Source: three-view drawing plus pictorial views. Frame: mm from the lowest corner of the part. Give positions to 0.01 mm unless a question says otherwise; leave off trailing zeros. Loops run counter-clockwise (first coordinate to the right, second up) from the corner with the lowest first, then second, coordinate; pieces in that order, holes last. Notation, with made-up numbers: (45.25, 87) - (87.25, 87) arc R17 ccw to (87.25, 120) - close; hole circle Ø4 at (54.5, -17.5). An arc over 180 degrees is marked (long way). Answer as a JSON object with one key per item and string values. Group by question number.
(1) Material intervals for L1, parallel to Z at x = 5, y = 2.75; L2, parallel to X at y = 2.1, z = 12, sorted ascending.
(2) Section query C-C (y = 2.8). Return loops of the section in (x, z), plus the area to 3 significant figures.
(3) Section query B-B (x = 5). Return loops of the section in (y, z).
(4) Section query A-A (z = 18). Return loops of the section in (x, y), plus the area to 3 significant figures.
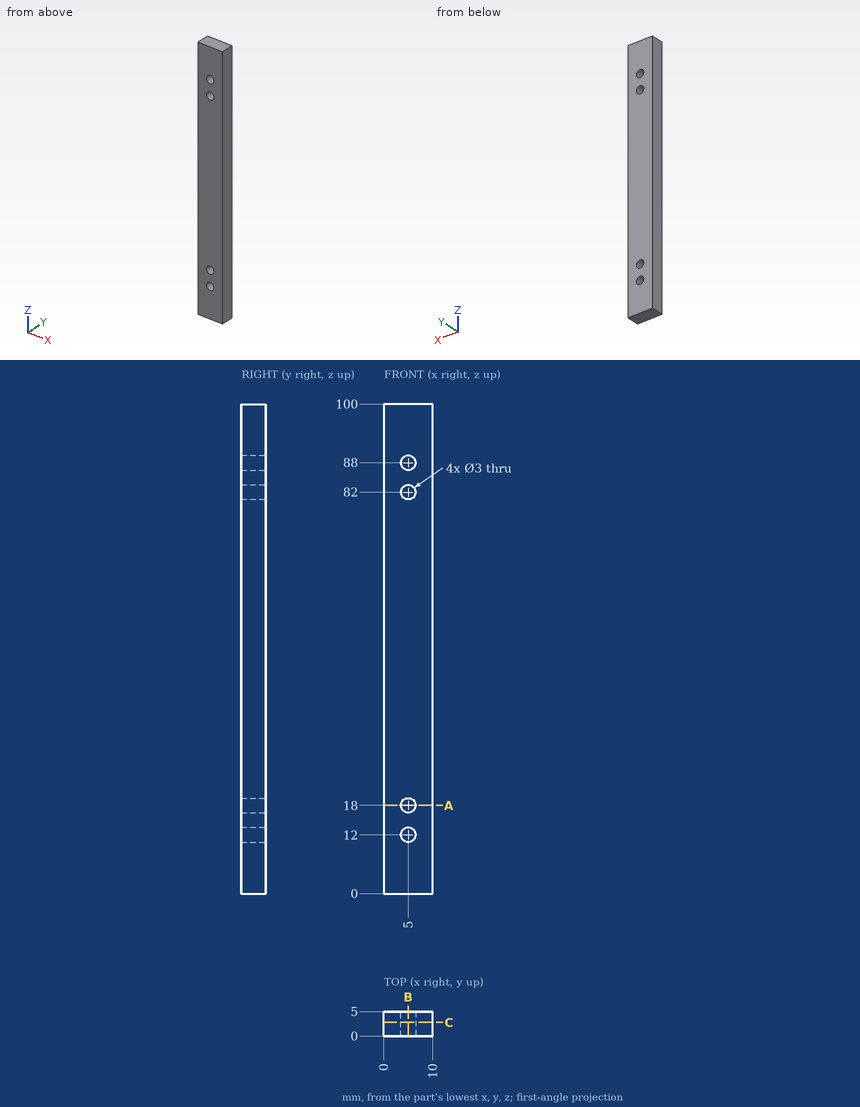
Recorded:
{
 "1": {"L1": "z = 0 to 10.5, 13.5 to 16.5, 19.5 to 80.5, 83.5 to 86.5, 89.5 to 100", "L2": "x = 0 to 3.5, 6.5 to 10"},
 "2": {"outline": "(0, 0) - (10, 0) - (10, 100) - (0, 100) - close; hole circle Ø3 at (5, 12); hole circle Ø3 at (5, 18); hole circle Ø3 at (5, 82); hole circle Ø3 at (5, 88)", "area": "972 mm^2"},
 "3": {"outline": "(0, 0) - (5, 0) - (5, 10.5) - (0, 10.5) - close; (0, 13.5) - (5, 13.5) - (5, 16.5) - (0, 16.5) - close; (0, 19.5) - (5, 19.5) - (5, 80.5) - (0, 80.5) - close; (0, 83.5) - (5, 83.5) - (5, 86.5) - (0, 86.5) - close; (0, 89.5) - (5, 89.5) - (5, 100) - (0, 100) - close"},
 "4": {"outline": "(0, 0) - (3.5, 0) - (3.5, 5) - (0, 5) - close; (6.5, 0) - (10, 0) - (10, 5) - (6.5, 5) - close", "area": "35.0 mm^2"}
}
